Check sheet for the modelled part. Datum: model origin and axes. Units: mm. A direction names the side the tool comes from. Give positions to 0.01 mm unless a question says otherwise; leave off trailing zeros. Write each loop counter-clockwise with the first axis right and the second up, starting at its lowest first coordinate (ties: lowest second). Pieces come first, ordered by that corner, then holes. Notation, with made-up numbers: M 6.5,42.5 L 48.5,42.5 A13 ccw 48.5,58.5 Z; hole C 36,0 d3. An arc over 180 degrees is marked long. Write item = value, one per line. Start each with the question number.
1) Scan lines: line 1 along X through (y, z) = (-4.5, -10.5); line 2 along Y through (x, z) = (75.5, -44); line 3 along Y through (x, z) = (87.5, -4.5). Record each from-to range of solid material in increasing order. Write a range as [from, to].
2) Mould release check, pull along X, two halves, no side actions. Record for faces 1 (the flat face through (58.763, -1, -3)), 2 (the flat face through (63.619, -1, -22)), 3 (the flat face through (85, -2, -42)): released by +X, released by -X, zero draft, split by the parting line, or undercut.
3) Go/stop test with flat-tipped pins: pin 1 (1.1 mm diameter, centred on x = 55, y = -1, fed in from +Z); pin 2 (0.6 mm diameter, centred on x = 61.5, y = -1, fed in from +Z); pin 3 (1 mm diameter, centred on y = -1.5, z = -47, fed in from +X). Record where each tip stops, or that it passes through.
4) Access from +Z, -Z, +X, -X, +Y, -Y to the whole of each face (thin tool, end or side, straight path). Record for faces 4 (the flat face through (66.502, -1, -22)), 5 (the flat face through (26, -1, -45)), 6 (the flat face through (40.025, -1, -31)), 7 (the flat face through (76, -2, -45)).
5) Cross-section at C-C, the plane y = -8.25. Record the cut outline in (x, z), plus the area to 3 significant figures.
6) Cross-section at B-B, the plane x = 85. Record the cut outline in (y, z).
7) Cross-section at D-D, the plane y = -1. Give the number of separate pieces and of enclosed holes in the cut face, plus the area to 3 significant figures.
8) Cross-section at A-A, the plane z = -31. Record the cut outline in (x, y), plus the area to 3 significant figures.
```python
from build123d import *

# Parameters (mm, degrees)
SKETCH1_W           = 100
SKETCH1_H           = 50
BOSS_EXTRUDE1_DEPTH = 5
SKETCH2_W           = 25
SKETCH2_H           = 50
BOSS_EXTRUDE2_DEPTH = 20
SKETCH3_W           = 13
SKETCH3_H           = 13
SKETCH3_W_2         = 20
SKETCH3_H_2         = 20
SKETCH3_W_3         = 4.5
SKETCH3_H_3         = 4.5
SKETCH3_W_4         = 1
SKETCH3_H_4         = 2.5
SKETCH3_W_5         = 6
SKETCH3_H_5         = 6
BOSS_EXTRUDE3_DEPTH = 2
SKETCH4_W           = 7
SKETCH4_H           = 40
BOSS_EXTRUDE4_DEPTH = 5


with BuildPart() as part:
    # Sketch1 → Boss-Extrude1 (new body)
    with BuildSketch(Plane(origin=(0, 0, 0), x_dir=(1, 0, 0), z_dir=(0, 1, 0))):
        with Locations((50, 25)):
            Rectangle(SKETCH1_W, SKETCH1_H)
    extrude(amount=BOSS_EXTRUDE1_DEPTH)

    # Sketch2 → Boss-Extrude2 (add)
    with BuildSketch(Plane.XZ):
        with Locations((10.5, -25)):
            Rectangle(SKETCH2_W, SKETCH2_H)
    extrude(amount=BOSS_EXTRUDE2_DEPTH)

    # Sketch3 → Boss-Extrude3 (add)
    with BuildSketch(Plane.XZ):
        with Locations((62.354538524, -13.5)):
            Rectangle(SKETCH3_W, SKETCH3_H)
        with Locations((58.854538524, -35)):
            Rectangle(SKETCH3_W_2, SKETCH3_H_2)
        with Locations((41.25, -44.75)):
            Rectangle(SKETCH3_W_3, SKETCH3_H_3)
        with Locations((36.230283198, -35.23329394)):
            Rectangle(SKETCH3_W_4, SKETCH3_H_4)
        with Locations((84.854538524, -15)):
            Rectangle(SKETCH3_W_5, SKETCH3_H_5)
        with Locations((84.854538524, -24)):
            Rectangle(SKETCH3_W_5, SKETCH3_H_5)
        with Locations((84.854538524, -33)):
            Rectangle(SKETCH3_W_5, SKETCH3_H_5)
        with Locations((84.854538524, -42)):
            Rectangle(SKETCH3_W_5, SKETCH3_H_5)
        with Locations((34.75, -44.75)):
            Rectangle(SKETCH3_W_3, SKETCH3_H_3)
        with Locations((28.25, -44.75)):
            Rectangle(SKETCH3_W_3, SKETCH3_H_3)
        with Locations((40.25, -36.25)):
            Rectangle(SKETCH3_W_3, SKETCH3_H_3)
        with Locations((28.25, -36.25)):
            Rectangle(SKETCH3_W_3, SKETCH3_H_3)
        with Locations((34.056841582, -35.253056661)):
            Rectangle(SKETCH3_W_4, SKETCH3_H_4)
        with Locations((32.169211896, -35.217412145)):
            Rectangle(SKETCH3_W_4, SKETCH3_H_4)
        with Locations((38.888023686, -30.936743788)):
            Rectangle(SKETCH3_W_4, SKETCH3_H_4)
        with Locations((40.525487338, -30.924614304)):
            Rectangle(SKETCH3_W_4, SKETCH3_H_4)
        with Locations((50.783834941, -47.406763186)):
            Rectangle(SKETCH3_W_4, SKETCH3_H_4)
        with Locations((52.26338259, -47.478555209)):
            Rectangle(SKETCH3_W_4, SKETCH3_H_4)
        with Locations((54.55859758, -47.386324582)):
            Rectangle(SKETCH3_W_4, SKETCH3_H_4)
        with Locations((56.374406059, -47.474432974)):
            Rectangle(SKETCH3_W_4, SKETCH3_H_4)
        with Locations((58.792603581, -47.659638141)):
            Rectangle(SKETCH3_W_4, SKETCH3_H_4)
        with Locations((61.225203353, -47.50620675)):
            Rectangle(SKETCH3_W_4, SKETCH3_H_4)
        with Locations((63.310020495, -47.607368237)):
            Rectangle(SKETCH3_W_4, SKETCH3_H_4)
        with Locations((65.19308114, -47.698739903)):
            Rectangle(SKETCH3_W_4, SKETCH3_H_4)
        with Locations((67.695813528, -47.480844473)):
            Rectangle(SKETCH3_W_4, SKETCH3_H_4)
        with Locations((51.620089841, -22.168837292)):
            Rectangle(SKETCH3_W_4, SKETCH3_H_4)
        with Locations((54.828135526, -22.168837292)):
            Rectangle(SKETCH3_W_4, SKETCH3_H_4)
        with Locations((57.621886299, -22.168837292)):
            Rectangle(SKETCH3_W_4, SKETCH3_H_4)
        with Locations((60.182498208, -22.168837292)):
            Rectangle(SKETCH3_W_4, SKETCH3_H_4)
        with Locations((64.118696459, -22.168837292)):
            Rectangle(SKETCH3_W_4, SKETCH3_H_4)
        with Locations((62.314527943, -22.168837292)):
            Rectangle(SKETCH3_W_4, SKETCH3_H_4)
        with Locations((67.001738379, -22.168837292)):
            Rectangle(SKETCH3_W_4, SKETCH3_H_4)
        with Locations((58.263095719, -3.26300702)):
            Rectangle(SKETCH3_W_4, SKETCH3_H_4)
        with Locations((60.618093401, -3.26300702)):
            Rectangle(SKETCH3_W_4, SKETCH3_H_4)
        with Locations((62.890151559, -3.26300702)):
            Rectangle(SKETCH3_W_4, SKETCH3_H_4)
        with Locations((65.395210185, -3.26300702)):
            Rectangle(SKETCH3_W_4, SKETCH3_H_4)
        with Locations((66.760195848, -3.26300702)):
            Rectangle(SKETCH3_W_4, SKETCH3_H_4)
    extrude(amount=BOSS_EXTRUDE3_DEPTH)

    # Sketch4 → Boss-Extrude4 (add)
    with BuildSketch(Plane.XZ):
        with Locations((76.072105727, -25)):
            Rectangle(SKETCH4_W, SKETCH4_H)
    extrude(amount=BOSS_EXTRUDE4_DEPTH)


solid = part.part
```
Reply:
q1.line_1 = [-2, 23], [72.57, 79.57]
q1.line_2 = [-5, 5]
q1.line_3 = [0, 5]
q2.face_1 = undercut
q2.face_2 = undercut
q2.face_3 = zero draft
q3.pin_1 = -20.92
q3.pin_2 = -7
q3.pin_3 = 68.2
q4.face_4 = -Y
q4.face_5 = +Z, -Z, -Y
q4.face_6 = +Z, -Y
q4.face_7 = -Z, +X, -Y
q5.outline = M -2,-50 L 23,-50 L 23,0 L -2,0 Z
q5.area = 1,250 mm2
q6.outline = M -2,-45 L 0,-45 L 0,-50 L 5,-50 L 5,0 L 0,0 L 0,-12 L -2,-12 L -2,-18 L 0,-18 L 0,-21 L -2,-21 L -2,-27 L 0,-27 L 0,-30 L -2,-30 L -2,-36 L 0,-36 L 0,-39 L -2,-39 Z
q7.separate_pieces = 39
q7.enclosed_holes = 0
q7.area = 2,410 mm2
q8.outline = M -2,-20 L 23,-20 L 23,0 L 38.39,0 L 38.39,-2 L 39.39,-2 L 39.39,0 L 40.03,0 L 40.03,-2 L 41.03,-2 L 41.03,0 L 48.85,0 L 48.85,-2 L 68.85,-2 L 68.85,0 L 72.57,0 L 72.57,-5 L 79.57,-5 L 79.57,0 L 81.85,0 L 81.85,-2 L 87.85,-2 L 87.85,0 L 100,0 L 100,5 L 0,5 L 0,0 L -2,0 Z
q8.area = 1,090 mm2
